The listing builds one solid part. Answer for the finished solid, in the listing's coordinates (mm). A direction names the side the tool comes from. Coordinates: 2 decimals unless noted, no trailing zeros. Write each loop counter-clockwise with the first axis right and the second up, starting at its lowest first coordinate (ties: lowest second). Pieces come first, ordered by that corner, then holes.
from build123d import *

# Parameters (mm, degrees)
SKETCH1_R           = 1.75
SKETCH1_R_2         = 5.1
SKETCH1_R_3         = 1.5
BOSS_EXTRUDE1_DEPTH = 3.5


with BuildPart() as part:
    # Sketch1 → Boss-Extrude1 (new body)
    with BuildSketch(Plane(origin=(0, 0, 0), x_dir=(1, 0, 0), z_dir=(0, 1, 0))):
        Polygon((-93.819210637, 7.180789363), (-11.819210637, 7.180789363), (-8, 11), (8, 11), (11.819210637, 7.180789363), (93.819210637, 7.180789363), (101.25, 14), (107.25, 14), (107.25, -14), (101.25, -14), (93.819210637, -7.180789363), (11.819210637, -7.180789363), (8, -11), (-8, -11), (-11.819210637, -7.180789363), (-93.819210637, -7.180789363), (-101.25, -14), (-107.25, -14), (-107.25, 14), (-101.25, 14), align=None)
        with Locations(Location((-8, 0, 0), (0, 0, 270))):
            Circle(SKETCH1_R, mode=Mode.SUBTRACT)
        with Locations(Location((8, 0, 0), (0, 0, 270))):
            Circle(SKETCH1_R, mode=Mode.SUBTRACT)
        with Locations(Location((0, 0, 0), (0, 0, 270))):
            Circle(SKETCH1_R_2, mode=Mode.SUBTRACT)
        with Locations(Location((-104.25, -11, 0), (0, 0, 90))):
            Circle(SKETCH1_R_3, mode=Mode.SUBTRACT)
        with Locations(Location((0, 8, 0), (0, 0, 270))):
            Circle(SKETCH1_R, mode=Mode.SUBTRACT)
        with Locations(Location((0, -8, 0), (0, 0, 90))):
            Circle(SKETCH1_R, mode=Mode.SUBTRACT)
        with Locations(Location((-104.25, 11, 0), (0, 0, 270))):
            Circle(SKETCH1_R_3, mode=Mode.SUBTRACT)
        with Locations(Location((104.25, 11, 0), (0, 0, 270))):
            Circle(SKETCH1_R_3, mode=Mode.SUBTRACT)
        with Locations(Location((104.25, -11, 0), (0, 0, 270))):
            Circle(SKETCH1_R_3, mode=Mode.SUBTRACT)
    extrude(amount=BOSS_EXTRUDE1_DEPTH)


solid = part.part
1. Find the intervals of material crossed by L1, parallel to Z at x = 104.25, y = 0.8; L2, parallel to X at y = 2, z = 0; L3, parallel to X at y = 1, z = 9, in increasing order.
Results found:
L1: z = -14 to -12.5, -9.5 to 9.5, 12.5 to 14
L2: x = -107.25 to -9.75, -6.25 to -5.1, 5.1 to 6.25, 9.75 to 107.25
L3: x = -107.25 to -95.8, -10 to -1.44, 1.44 to 10, 95.8 to 107.25
2. Section C-C on x = -85 is taken. Give the vertices of the cut face in (y, z).
Results found:
outline: (0, -7.18) - (3.5, -7.18) - (3.5, 7.18) - (0, 7.18) - close
3. A tool of negligible diameter and unlimited length cuts with its end or side. For faces 1 (the flat face through (-10, 2, -9)), 2 (the flat face through (-104, 2, -14)), 3 (the flat face through (0, 2, 11)), from which of +Z, -Z, +X, -X, +Y, -Y can it reach the whole face along a straight path? Write none if from no direction.
Results found:
face 1: -Z, +Y, -Y
face 2: -Z, +X, -X, +Y, -Y
face 3: +Z, +Y, -Y
4. For a pull along Z with two mould halves and no side action, classify faces 4 (the flat face through (10, 2, -9)), 5 (the cylindrical face through (1.532, 1.726, 4.864)), 6 (the flat face through (-10, 2, 9)) as pulls with the +Z half, pulls with the -Z half, needs draft (parallel to the pull), parting line crosses it, or undercut.
Results found:
face 4: pulls with the -Z half
face 5: undercut
face 6: pulls with the +Z half
5. Section B-B on x = 0 is taken. Give the vertices of the cut face in (y, z), then the cut area to 3 significant figures.
Results found:
outline: (0, -11) - (3.5, -11) - (3.5, -9.75) - (0, -9.75) - close; (0, -6.25) - (3.5, -6.25) - (3.5, -5.1) - (0, -5.1) - close; (0, 5.1) - (3.5, 5.1) - (3.5, 6.25) - (0, 6.25) - close; (0, 9.75) - (3.5, 9.75) - (3.5, 11) - (0, 11) - close
area: 16.8 mm2
6. Section A-A on y = 0.9 is taken. State how many separate pieces and enclosed holes the cut face has, then the cut area to 3 significant figures.
Results found:
separate pieces: 1
enclosed holes: 9
area: 3,350 mm2
7. Flat-ended cylindrical pins translate along their axes: P1, Ø1.8, axis at x = 2, y = 2, coming from the +Z side; P2, Ø1, axis at x = 2, y = 1.5, coming from the -Z side. Find the tip coordinate at first contact, or state that the pin passes through.
Results found:
P1: stops at z = 11
P2: stops at z = -11
